Check sheet for the drawn part. Datum: minimum x, y, z corner. Units: mm. Round coordinates to 2 decimals unless told otherwise and drop trailing zeros. Write each loop counter-clockwise with the first axis right and the second up, starting at its lowest first coordinate (ties: lowest second). Pieces come first, ordered by that corner, then holes. Notation, with made-up numbers: (48, 30.25) - (89, 30.25) arc R25 cw to (89, 56.25) - close; hole circle Ø2 at (22.25, 59.25). An arc over 180 degrees is marked (long way). Answer as a JSON object with one key per item and string values.
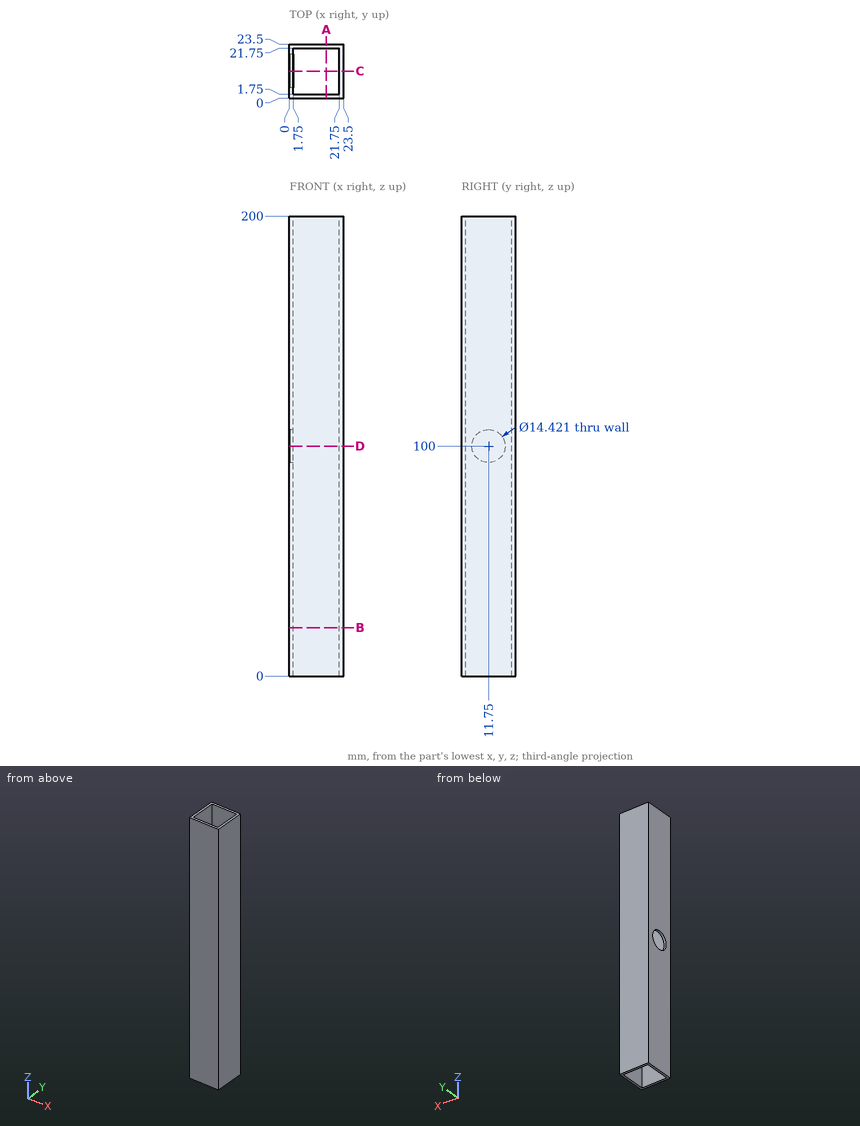
Q1. Section check C-C, the plane y = 11.75. Record the cut outline in (x, z).
Geometry check:
{"outline": "(0, 0) - (1.75, 0) - (1.75, 92.79) - (0, 92.79) - close; (0, 107.21) - (1.75, 107.21) - (1.75, 200) - (0, 200) - close; (21.75, 0) - (23.5, 0) - (23.5, 200) - (21.75, 200) - close"}
Q2. Section check B-B, the plane z = 21. Record the cut outline in (x, y).
Geometry check:
{"outline": "(0, 0) - (23.5, 0) - (23.5, 23.5) - (0, 23.5) - close; hole (1.75, 1.75) - (21.75, 1.75) - (21.75, 21.75) - (1.75, 21.75) - close"}
Q3. Section check D-D, the plane z = 100. Record the cut outline in (x, y), then the cut area to 3 significant figures.
Geometry check:
{"outline": "(0, 0) - (23.5, 0) - (23.5, 23.5) - (0, 23.5) - (0, 18.96) - (1.75, 18.96) - (1.75, 21.75) - (21.75, 21.75) - (21.75, 1.75) - (1.75, 1.75) - (1.75, 4.54) - (0, 4.54) - close", "area": "127 mm2"}
Q4. Material ranges on line 1 along Y through (x, z) = (21.5, 151.5); line 2 along Y through (x, z) = (1.25, 100), recorded low to high. Write a range as [from, to].
Geometry check:
{"line 1": "y = [0, 1.75], [21.75, 23.5]", "line 2": "y = [0, 4.54], [18.96, 23.5]"}
Q5. Gauge pin test, flat end, axial feed: P1, Ø1.5, axis at x = 4.5, z = 79.5, coming from the -Y side. Record the tip position at first contact, or that the pin passes through.
Geometry check:
{"P1": "stops at y = 0"}
Q6. Section check A-A, the plane x = 16. Record the cut outline in (y, z).
Geometry check:
{"outline": "(0, 0) - (1.75, 0) - (1.75, 200) - (0, 200) - close; (21.75, 0) - (23.5, 0) - (23.5, 200) - (21.75, 200) - close"}
